Answer from the drawing. Dimensions are ordinates in mm from the lowest x, y and z of the part. A direction names the side the tool comes from. Round coordinates to 2 decimals unless told otherwise and drop trailing zeros. Order: outer loops, then holes, each group sorted by start corner. A loop starts at its lowest first (then second) coordinate and runs counter-clockwise, first axis right, second up. Notation, with made-up numbers: M 19.5,13.25 L 24.5,13.25 A29 ccw 24.5,40.25 Z; hole C 47.25,11.25 d3. An arc over 180 degrees is marked long. Answer as a JSON object with one key per item and string values. Group by question number.
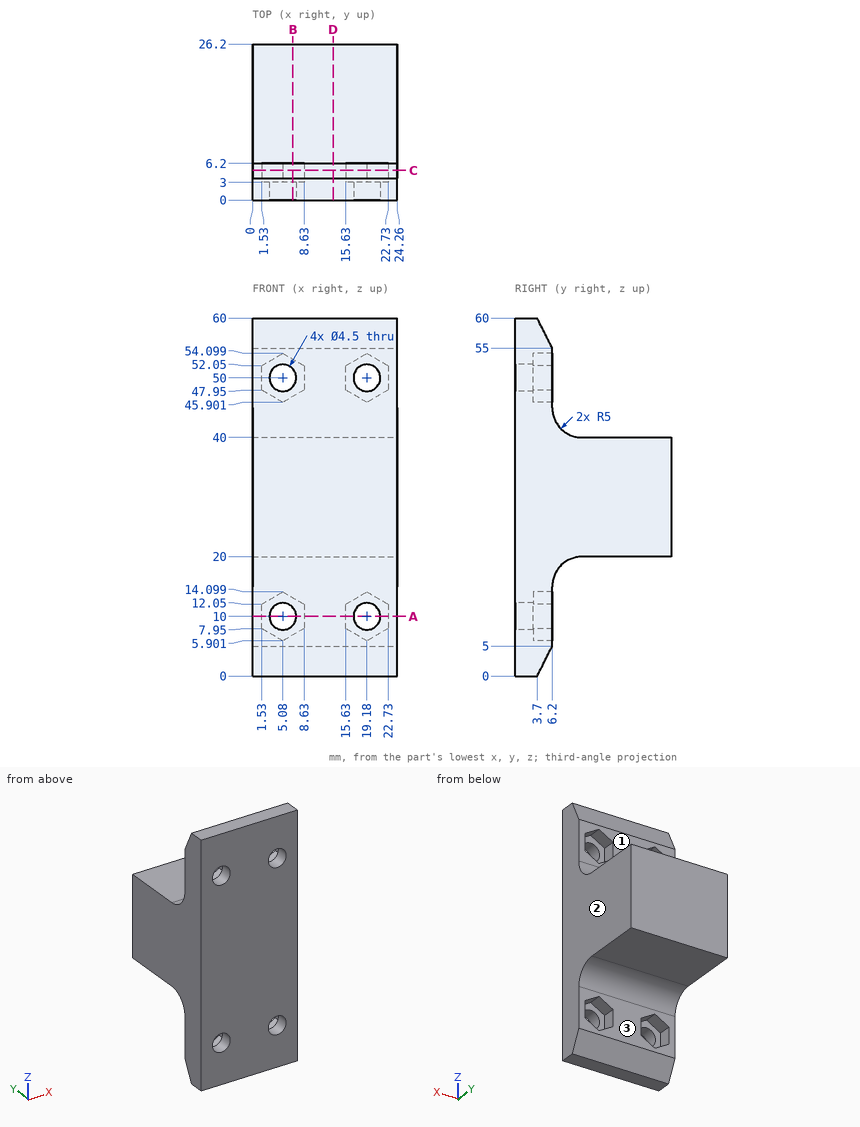
Item 1: Find section B-B (x = 6.75). Give the vertices of the cut face in (y, z) (1 decimal), and give its area (3 significant figures).
Item 2: Consider L1, parallel to X at y = 5.5, z = 49.5; L2, parallel to X at y = 2.1, z = 50; L3, parallel to Z at x = 7.75, y = 4 (1 decimal). Determine where each line is inside the solid, lowest interval first.
Item 3: Find section C-C (y = 5). Give the vertices of the cut face in (x, z).
Item 4: Each of these flat-tipped pins is pushed along its axis until it touches: pin 1 (8 mm diameter, centred on x = 13.5, z = 49, fed in from +Y); pin 2 (1.5 mm diameter, centred on x = 8, y = 4.5, fed in from +Z); pin 3 (6 mm diameter, centred on x = 9, y = 15, fed in from -Z); pin 4 (2 mm diameter, centred on x = 4, z = 50, fed in from +Y). Where does it stop, or does it pass through?
Item 5: Find section A-A (z = 10). Give the vertices of the cut face in (x, y).
Item 6: A tool of negligible diameter and unlimited length cuts with its end or side. For the marked faces 1, 2 and 3, from which of +Z, -Z, +X, -X, +Y, -Y can it reach the whole face along a straight path? Write none if from no direction.
Item 7: Find section D-D (x = 13.5). Give the vertices of the cut face in (y, z).
Responses:
{
 "1": {"outline": "M 0,0 L 3.7,0 L 6.2,5 L 6.2,6.9 L 3,6.9 L 3,8.5 L 0,8.5 Z; M 0,11.5 L 3,11.5 L 3,13.1 L 6.2,13.1 L 6.2,15 A5 cw 11.2,20 L 26.2,20 L 26.2,40 L 11.2,40 A5 cw 6.2,45 L 6.2,46.9 L 3,46.9 L 3,48.5 L 0,48.5 Z; M 0,51.5 L 3,51.5 L 3,53.1 L 6.2,53.1 L 6.2,55 L 3.7,60 L 0,60 Z", "area": "712 mm^2"},
 "2": {"L1": "x = 0 to 1.53, 8.63 to 15.63, 22.73 to 24.26", "L2": "x = 0 to 2.83, 7.33 to 16.93, 21.43 to 24.26", "L3": "z = 0.6 to 7.4, 12.6 to 47.4, 52.6 to 59.4"},
 "3": {"outline": "M 0,2.6 L 24.26,2.6 L 24.26,57.4 L 0,57.4 Z; hole M 1.53,7.95 L 5.08,5.9 L 8.63,7.95 L 8.63,12.05 L 5.08,14.1 L 1.53,12.05 Z; hole M 1.53,47.95 L 5.08,45.9 L 8.63,47.95 L 8.63,52.05 L 5.08,54.1 L 1.53,52.05 Z; hole M 15.63,7.95 L 19.18,5.9 L 22.73,7.95 L 22.73,12.05 L 19.18,14.1 L 15.63,12.05 Z; hole M 15.63,47.95 L 19.18,45.9 L 22.73,47.95 L 22.73,52.05 L 19.18,54.1 L 15.63,52.05 Z"},
 "4": {"pin 1": "stops at y = 6.2", "pin 2": "stops at z = 59.9", "pin 3": "stops at z = 20", "pin 4": "passes through"},
 "5": {"outline": "M 0,0 L 2.83,0 L 2.83,3 L 1.53,3 L 1.53,6.2 L 0,6.2 Z; M 7.33,0 L 16.93,0 L 16.93,3 L 15.63,3 L 15.63,6.2 L 8.63,6.2 L 8.63,3 L 7.33,3 Z; M 21.43,0 L 24.26,0 L 24.26,6.2 L 22.73,6.2 L 22.73,3 L 21.43,3 Z"},
 "6": {"face 1": "+Z, +X, -X, +Y", "face 2": "+Z, -Z, +X, +Y, -Y", "face 3": "-Z, +X, -X, +Y"},
 "7": {"outline": "M 0,0 L 3.7,0 L 6.2,5 L 6.2,15 A5 cw 11.2,20 L 26.2,20 L 26.2,40 L 11.2,40 A5 cw 6.2,45 L 6.2,55 L 3.7,60 L 0,60 Z"}
}
